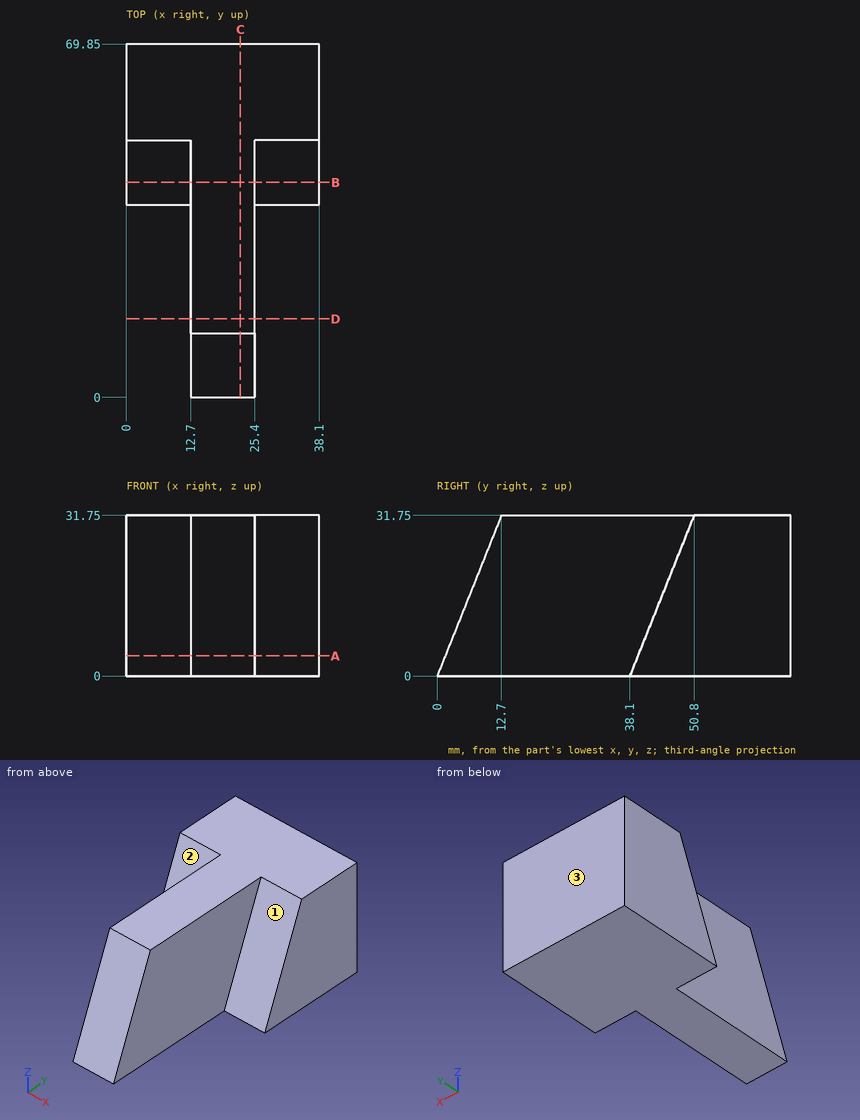
For this review, use the dimensioned drawing (mm, ordinates from the lowest corner) and the shaded views. A direction names the side the tool comes from. Coordinates: 2 decimals unless noted, no trailing zeros. Order: outer loops, then holes, each group sorted by start corner. A loop starts at its lowest first (then second) coordinate and runs counter-clockwise, first axis right, second up. Notation, with made-up numbers: (31.5, 16.5) - (86.5, 16.5) arc R16 cw to (86.5, 24.5) - close; hole circle Ø2 at (-15, 19). An arc over 180 degrees is marked (long way). Answer in a Markdown table with one row per item.
(1) Consider section C-C on x = 22.5. State the section outline as (y, z) points.
Checked values:
| item | result |
|---|---|
| outline | (0, 0) - (69.85, 0) - (69.85, 31.75) - (12.7, 31.75) - close |
(2) Wall thickness on line 1 along X through (y, z) = (15, 29); line 2 along Y through (x, z) = (19.5, 14); line 3 along Y through (x, z) = (5.5, 27.5): over which ranges is each line inside the solid? List them lowest first. Write a range as from..to.
Checked values:
| item | result |
|---|---|
| line 1 | 12.7..25.4 |
| line 2 | 5.6..69.85 |
| line 3 | 49.1..69.85 |
(3) For the marked faces 1, 2 and 3, list the 3-axis set-ups (+Z, -Z, +X, -X, +Y, -Y) from which the entire face can be reached by the end or side of a thin tool; tool diameter is ignored.
Checked values:
| item | result |
|---|---|
| face 1 | +Z, +X, -Y |
| face 2 | +Z, -X, -Y |
| face 3 | +Z, -Z, +X, -X, +Y |
(4) Clearance check with flat-ended pins moving along their axes: pin 1 (16 mm diameter, centred on y = 23, z = 19, fed in from +X); pin 2 (6 mm diameter, centred on x = 32, z = 27.5, fed in from -Y); pin 3 (10 mm diameter, centred on x = 7, y = 20, fed in from +Z). State where each tip first meets the part, or that it passes through.
Checked values:
| item | result |
|---|---|
| pin 1 | x = 25.4 |
| pin 2 | y = 47.9 |
| pin 3 | through |
(5) Consider section D-D on y = 15.5. State the section outline as (x, z) points, plus the area to 3 significant figures.
Checked values:
| item | result |
|---|---|
| outline | (12.7, 0) - (25.4, 0) - (25.4, 31.75) - (12.7, 31.75) - close |
| area | 403 mm^2 |
(6) Consider section B-B on y = 42.5. State the section outline as (x, z) points, plus the area to 3 significant figures.
Checked values:
| item | result |
|---|---|
| outline | (0, 0) - (38.1, 0) - (38.1, 11) - (25.4, 11) - (25.4, 31.75) - (12.7, 31.75) - (12.7, 11) - (0, 11) - close |
| area | 683 mm^2 |
(7) Consider section A-A on z = 4. State the section outline as (x, y) points.
Checked values:
| item | result |
|---|---|
| outline | (0, 39.7) - (12.7, 39.7) - (12.7, 1.6) - (25.4, 1.6) - (25.4, 39.7) - (38.1, 39.7) - (38.1, 69.85) - (0, 69.85) - close |
